Read the model definition and answer for the solid it produces. Units are mm, in the model's axes. Face numbers are marked on the shaded views. Give positions to 0.01 mm unless a question says otherwise; leave off trailing zeros. Loops run counter-clockwise (first coordinate to the right, second up) from the corner with the lowest first, then second, coordinate; pieces in that order, holes last. Notation, with made-up numbers: (18.25, 48) - (71.25, 48) arc R19 cw to (71.25, 71) - close; hole circle Ø1 at (84.5, -23.5). An arc over 180 degrees is marked (long way). Write item = value, one per line.
```python
from build123d import *

# Parameters (mm, degrees)
SKETCH1_W           = 15
SKETCH1_H           = 88
BOSS_EXTRUDE1_DEPTH = 3
SKETCH2_W           = 15
SKETCH2_H           = 5
BOSS_EXTRUDE2_DEPTH = 10
SKETCH3_W           = 15
SKETCH3_H           = 5
BOSS_EXTRUDE3_DEPTH = 10


with BuildPart() as part:
    # Sketch1 → Boss-Extrude1 (new body, symmetric)
    with BuildSketch(Plane.XY):
        with Locations((0, 44)):
            Rectangle(SKETCH1_W, SKETCH1_H)
    extrude(amount=BOSS_EXTRUDE1_DEPTH, both=True)

    # Sketch2 → Boss-Extrude2 (add)
    with BuildSketch(Plane.XY):
        with Locations((0, 2.5)):
            Rectangle(SKETCH2_W, SKETCH2_H)
    extrude(amount=BOSS_EXTRUDE2_DEPTH)

    # Sketch3 → Boss-Extrude3 (add)
    with BuildSketch(Plane.XY):
        with Locations((0, 85.5)):
            Rectangle(SKETCH3_W, SKETCH3_H)
    extrude(amount=BOSS_EXTRUDE3_DEPTH)


solid = part.part
```
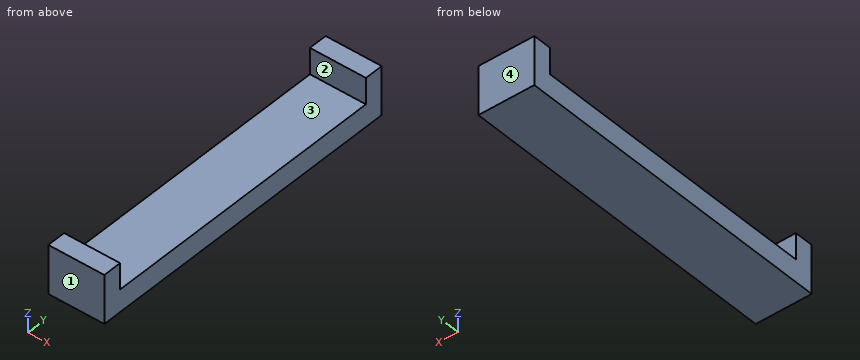
1) Find the intervals of material crossed by probe 1 along Y at (x, z) = (3, 9.25); probe 2 along Z at (x, y) = (-4.5, 72), in increasing order.
Output:
probe_1 = 0 to 5, 83 to 88
probe_2 = -3 to 3
2) Each of these flat-tipped pins is pushed along its axis until it touches: P1, Ø1, axis at x = 5.5, y = 72, coming from the +Z side; P2, Ø2, axis at x = 0.5, z = 7.5, coming from the -Y side. Where does it stop, or does it pass through?
Output:
P1 = 3
P2 = 0
3) A cutting plane is placed at A-A on z = 5.5. Determine the outline of the cut face in (x, y), then the cut area to 3 significant figures.
Output:
outline = (-7.5, 0) - (7.5, 0) - (7.5, 5) - (-7.5, 5) - close; (-7.5, 83) - (7.5, 83) - (7.5, 88) - (-7.5, 88) - close
area = 150 mm²
4) A cutting plane is placed at B-B on x = -3. Determine the outline of the cut face in (y, z).
Output:
outline = (0, -3) - (88, -3) - (88, 10) - (83, 10) - (83, 3) - (5, 3) - (5, 10) - (0, 10) - close
5) A cutting plane is placed at C-C on y = 29. Determine the outline of the cut face in (x, z).
Output:
outline = (-7.5, -3) - (7.5, -3) - (7.5, 3) - (-7.5, 3) - close
6) The mould has two halves that part along Y. Classify the marked faces 1, 2, 3 and 4: pulls with the +Y half, pulls with the -Y half, needs draft (parallel to the pull), parting line crosses it, or undercut.
Output:
face_1 = pulls with the -Y half
face_2 = undercut
face_3 = undercut
face_4 = pulls with the +Y half
